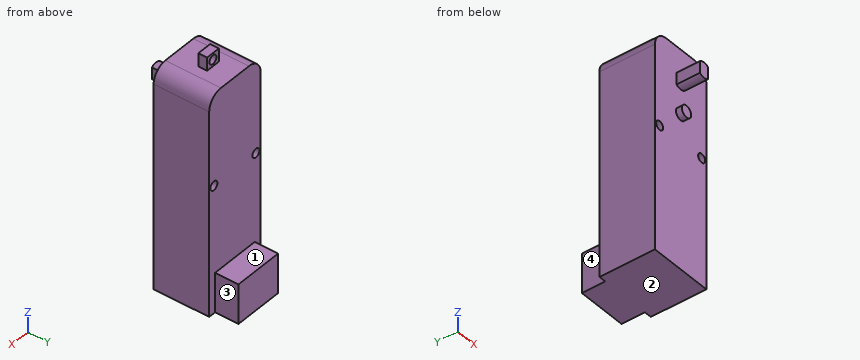
```python
from build123d import *

# Parameters (mm, degrees)
SKETCH1_W               = 22
SKETCH1_H               = 75
BOSS_EXTRUDE1_DEPTH     = 19
SKETCH2_W               = 17
SKETCH2_H               = 13.5
BOSS_EXTRUDE2_DEPTH     = 8
FILLET1_R               = 5
SKETCH4_R               = 2.65
BOSS_EXTRUDE3_DEPTH     = 8
CUT_EXTRUDE1_DEPTH      = 83.692200358
CUT_EXTRUDE1_DEPTH_BACK = 83.692200358
SKETCH5_R               = 1.5
SKETCH6_R               = 2
SKETCH6_R_2             = 2.65
BOSS_EXTRUDE4_DEPTH     = 2
CUT_EXTRUDE2_DEPTH      = 86.638776264
CUT_EXTRUDE2_DEPTH_BACK = 8
SKETCH8_W               = 5
SKETCH8_H               = 3
BOSS_EXTRUDE5_DEPTH     = 4.5
SKETCH9_R               = 1.5
CUT_EXTRUDE3_DEPTH      = 3


with BuildPart() as part:
    # Sketch1 → Boss-Extrude1 (new body)
    with BuildSketch(Plane(origin=(0, 0, 0), x_dir=(1, 0, 0), z_dir=(0, 1, 0))):
        with Locations((11, 37.5)):
            Rectangle(SKETCH1_W, SKETCH1_H)
    extrude(amount=BOSS_EXTRUDE1_DEPTH)

    # Sketch2 → Boss-Extrude2 (add)
    with BuildSketch(Plane(origin=(0, 19, 0), x_dir=(1, 0, 0), z_dir=(0, 1, 0))):
        with Locations((11, 68.25)):
            Rectangle(SKETCH2_W, SKETCH2_H)
    extrude(amount=BOSS_EXTRUDE2_DEPTH)

    # Fillet1
    fillet1_edges = [part.edges().sort_by_distance(p)[0] for p in [
        (22, 9.5, 0),
        (0, 9.5, 0),
    ]]
    fillet(fillet1_edges, radius=FILLET1_R)

    # Sketch4 → Boss-Extrude3 (add)
    with BuildSketch(Plane.XZ):
        with Locations(Location((11, -11, 0), (0, 0, 270))):
            Circle(SKETCH4_R)
    extrude(amount=BOSS_EXTRUDE3_DEPTH)

    # Sketch5 → Cut-Extrude1 (cut, two sides: drawn at the far end of the back side and taken through both)
    with BuildSketch(Plane.XZ.offset(-CUT_EXTRUDE1_DEPTH_BACK)):
        with Locations(Location((20, -31.5, 0), (0, 0, 270))):
            Circle(SKETCH5_R)
        with Locations(Location((2, -31.5, 0), (0, 0, 270))):
            Circle(SKETCH5_R)
    extrude(amount=CUT_EXTRUDE1_DEPTH + CUT_EXTRUDE1_DEPTH_BACK, mode=Mode.SUBTRACT)

    # Sketch6 → Boss-Extrude4 (add)
    with BuildSketch(Plane.XZ):
        with Locations(Location((11, -22.15, 0), (0, 0, 270))):
            Circle(SKETCH6_R)
        with Locations(Location((11, -11, 0), (0, 0, 270))):
            Circle(SKETCH6_R_2)
    extrude(amount=BOSS_EXTRUDE4_DEPTH)

    # Sketch7 → Cut-Extrude2 (cut, two sides: drawn at the far end of the back side and taken through both)
    with BuildSketch(Plane.XZ.offset(8).offset(-CUT_EXTRUDE2_DEPTH_BACK)):
        with BuildLine():
            Line((12.75, -9.010025126), (12.75, -12.989974874))
            ThreePointArc((12.75, -12.989974874), (13.65, -11), (12.75, -9.010025126))
        make_face()
        with BuildLine():
            Line((9.25, -9.010025126), (9.25, -12.989974874))
            ThreePointArc((9.25, -12.989974874), (8.35, -11), (9.25, -9.010025126))
        make_face()
    extrude(amount=CUT_EXTRUDE2_DEPTH + CUT_EXTRUDE2_DEPTH_BACK, mode=Mode.SUBTRACT)

    # Sketch8 → Boss-Extrude5 (add)
    with BuildSketch(Plane.XY):
        with Locations((11, 10)):
            Rectangle(SKETCH8_W, SKETCH8_H)
    extrude(amount=BOSS_EXTRUDE5_DEPTH)

    # Sketch9 → Cut-Extrude3 (cut)
    with BuildSketch(Plane(origin=(0, 11.5, 0), x_dir=(1, 0, 0), z_dir=(0, 1, 0))):
        with Locations(Location((11, -2.25, 0), (0, 0, 180))):
            Circle(SKETCH9_R)
    extrude(amount=-CUT_EXTRUDE3_DEPTH, mode=Mode.SUBTRACT)


solid = part.part
```
The listing builds one solid part. Answer for the finished solid, in the listing's coordinates (mm). Face numbers are marked on the shaded views. A direction names the side the tool comes from. Coordinates: 2 decimals unless noted, no trailing zeros. Loops run counter-clockwise (first coordinate to the right, second up) from the corner with the lowest first, then second, coordinate; pieces in that order, holes last. Notation, with made-up numbers: (-24, -16) - (3, -16) arc R23 ccw to (3, 14) - close; hole circle Ø10 at (10, 67.5). An arc over 180 degrees is marked (long way). Use a Markdown table: item, result. Add a question column.
1) The part is cut by section B-B, the plane y = 5.5. Give the vertices of the cut face in (x, z), and give its area (3 significant figures).
2) The part is cut by section D-D, the plane z = -22.15. Give the vertices of the cut face in (x, y), and give its area (3 significant figures).
3) The part is cut by section A-A, the plane z = -31.5. Give the vertices of the cut face in (x, y).
4) For the marked faces 1, 2, 3 and 4, determine the directions among +Z, -Z, +X, -X, +Y, -Y from which every point of the face is accessible in a straight line to the end or side of a thin tool.
5) The part is cut by section C-C, the plane x = 11. Give the vertices of the cut face in (y, z), and give its area (3 significant figures).
6) Given pin 1 (11 mm diameter, centred on x = 14.5, z = -42.5, fed in from +Y); pin 2 (2.5 mm diameter, centred on x = 11, z = 2.25, fed in from -Y); pin 3 (4 mm diameter, centred on x = 12.5, y = 23, fed in from +Z); pin 4 (3.5 mm diameter, centred on x = 2, z = -31.5, fed in from -Y), each flat-ended and moving along its own axis, determine where each tip first touches the part or whether it passes through.
7) Find the intervals of material crossed by line 1 (X direction, y = 5, z = -31.5); line 2 (X direction, y = 14, z = -31); line 3 (Y direction, x = 8.5, z = -37), in increasing order.
Here are the results:
| question | item | result |
|---|---|---|
| 1 | outline | (0, -75) - (22, -75) - (22, -5) arc R5 ccw to (17, 0) - (5, 0) arc R5 ccw to (0, -5) - close; hole circle Ø3 at (2, -31.5); hole circle Ø3 at (20, -31.5) |
| 1 | area | 1,630 mm^2 |
| 2 | outline | (0, 0) - (9, 0) - (9, -2) - (13, -2) - (13, 0) - (22, 0) - (22, 19) - (0, 19) - close |
| 2 | area | 426 mm^2 |
| 3 | outline | (0, 0) - (0.5, 0) - (0.5, 19) - (0, 19) - close; (3.5, 0) - (18.5, 0) - (18.5, 19) - (3.5, 19) - close; (21.5, 0) - (22, 0) - (22, 19) - (21.5, 19) - close |
| 4 | face 1 | +Z, +X, -X, +Y |
| 4 | face 2 | -Z, +X, -X, +Y, -Y |
| 4 | face 3 | +Z, -Z, +X, +Y |
| 4 | face 4 | +Z, -Z, -X, +Y |
| 5 | outline | (-8, -13.65) - (0, -13.65) - (0, -20.15) - (-2, -20.15) - (-2, -24.15) - (0, -24.15) - (0, -75) - (27, -75) - (27, -61.5) - (19, -61.5) - (19, 0) - (11.5, 0) - (11.5, 0.75) - (8.5, 0.75) - (8.5, 0) - (0, 0) - (0, -8.35) - (-8, -8.35) - close; (8.5, 3.75) - (11.5, 3.75) - (11.5, 4.5) - (8.5, 4.5) - close |
| 5 | area | 1,590 mm^2 |
| 6 | pin 1 | stops at y = 19 |
| 6 | pin 2 | passes through |
| 6 | pin 3 | stops at z = -61.5 |
| 6 | pin 4 | stops at y = 0 |
| 7 | line 1 | x = 0 to 0.5, 3.5 to 18.5, 21.5 to 22 |
| 7 | line 2 | x = 0 to 0.59, 3.41 to 18.59, 21.41 to 22 |
| 7 | line 3 | y = 0 to 19 |
